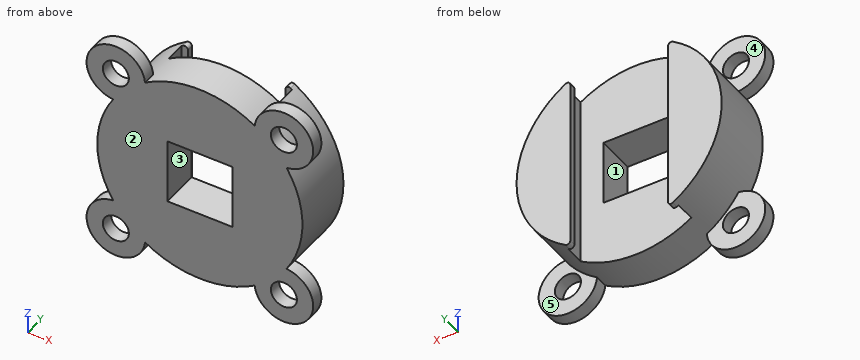
```python
from build123d import *

# Parameters (mm, degrees)
CYLINDER008_R         = 15.75
CYLINDER008_DEPTH     = 10
CYLINDER009_R         = 4.5
CYLINDER009_DEPTH     = 2
POLARPATTERN002_COUNT = 4
CYLINDER010_R         = 2
CYLINDER010_DEPTH     = 2
POLARPATTERN003_COUNT = 4
BOX001_W              = 10
BOX001_H              = 10
BOX001_DEPTH          = 10
BOX003_W              = 32.5
BOX003_H              = 17
BOX003_DEPTH          = 3.1
BOX004_W              = 32.5
BOX004_H              = 15
BOX004_DEPTH          = 1
FILLET005_R           = 0.5


with BuildPart() as part:
    # Cylinder008 → Cylinder008 (join)
    with BuildSketch(Plane(origin=(0, 0, 0), x_dir=(-1, 0, 0), z_dir=(0, 1, 0))):
        Circle(CYLINDER008_R)
    extrude(amount=CYLINDER008_DEPTH)

    # Cylinder009 → Cylinder009 (join)
    with BuildSketch(Plane(origin=(12.904699, 0, -12.904699), x_dir=(0, 0, -1), z_dir=(0, 1, 0))):
        Circle(CYLINDER009_R)
    cylinder009 = extrude(amount=CYLINDER009_DEPTH)

    # PolarPattern002: Cylinder009 ×4 about axis
    polarpattern002_axis = Axis((0, 0, 0), (0, 1, 0))
    for i in range(1, POLARPATTERN002_COUNT):
        add(cylinder009.rotate(polarpattern002_axis, i * 360 / POLARPATTERN002_COUNT))

    # Cylinder010 → Cylinder010 (cut)
    with BuildSketch(Plane(origin=(12.904699, 0, 12.904699), x_dir=(0, 0, -1), z_dir=(0, 1, 0))):
        Circle(CYLINDER010_R)
    cylinder010 = extrude(amount=CYLINDER010_DEPTH, mode=Mode.SUBTRACT)

    # PolarPattern003: Cylinder010 ×4 about axis
    polarpattern003_axis = Axis((0, 0, 0), (0, 1, 0))
    for i in range(1, POLARPATTERN003_COUNT):
        add(cylinder010.rotate(polarpattern003_axis, i * 360 / POLARPATTERN003_COUNT), mode=Mode.SUBTRACT)

    # Box001 → Box001 (cut)
    with BuildSketch(Plane(origin=(5, 0, -5), x_dir=(-1, 0, 0), z_dir=(0, 1, 0))):
        with Locations((5, 5)):
            Rectangle(BOX001_W, BOX001_H)
    extrude(amount=BOX001_DEPTH, mode=Mode.SUBTRACT)

    # Box003 → Box003 (cut)
    with BuildSketch(Plane(origin=(-8.5, 9, 16.25), x_dir=(0, 0, -1), z_dir=(0, -1, 0))):
        with Locations((16.25, 8.5)):
            Rectangle(BOX003_W, BOX003_H)
    extrude(amount=BOX003_DEPTH, mode=Mode.SUBTRACT)

    # Box004 → Box004 (cut)
    with BuildSketch(Plane(origin=(-7.5, 10, 16.25), x_dir=(0, 0, -1), z_dir=(0, -1, 0))):
        with Locations((16.25, 7.5)):
            Rectangle(BOX004_W, BOX004_H)
    extrude(amount=BOX004_DEPTH, mode=Mode.SUBTRACT)

    # Fillet005
    fillet005_edges = [part.edges().sort_by_distance(p)[0] for p in [
        (-7.5, 9.5, -13.849639),
        (7.5, 9.5, 13.849639),
        (-7.5, 9.5, 13.849639),
        (7.5, 9.5, -13.849639),
    ]]
    fillet(fillet005_edges, radius=FILLET005_R)


solid = part.part
```
Source: CAD feature listing. Evaluate the final solid. Frame: model axes, mm. Face numbers are marked on the shaded views. A direction names the side the tool comes from. Round coordinates to 2 decimals unless told otherwise and drop trailing zeros. Loops run counter-clockwise (first coordinate to the right, second up) from the corner with the lowest first, then second, coordinate; pieces in that order, holes last.
1. Mould query, pull axis Z, two halves, no side actions, for the marked faces 1 and 2. Classes: released by +Z, released by -Z, zero draft, split by the parting line, or undercut.
2. Ray query, L1, parallel to Y at x = -8, z = 11; L2, parallel to X at y = 1.75, z = -13.5; L3, parallel to X at y = 5.5, z = -2. Return the intervals inside material, ascending.
3. Access query for the marked faces 3, 4 and 5. Directions: +Z, -Z, +X, -X, +Y, -Y. A direction counts if a zero-diameter tool reaches every point of the face in a straight line with its end or side. Return the directions, or none.
4. Section query D-D on z = -11.5. Output: boundary loops of the cut face in (x, y), and give its area (3 significant figures).
5. Section query A-A on x = 0. Output: boundary loops of the cut face in (y, z).
6. Section query B-B on z = 0. Output: boundary loops of the cut face in (x, y).
7. Contact query for flat-ended pins moving along their axis: pin 1 (0.8 mm diameter, centred on y = 9.5, z = 0.5, fed in from -X); pin 2 (4.5 mm diameter, centred on x = 12.5, z = -13, fed in from +Y); pin 3 (1 mm diameter, centred on y = 8.5, z = 12, fed in from +X). Output: stop coordinate, or through.
8. Section query C-C on y = 8.5. Output: boundary loops of the cut face in (x, z), and give its area (3 significant figures).
Answers below:
1. face 1: undercut
1. face 2: zero draft
2. L1: y = 0 to 5.9, 9 to 10
2. L2: x = -17.37 to -14.81, -11 to -8.44, -8.11 to 8.11, 8.44 to 11, 14.81 to 17.37
2. L3: x = -15.62 to -5, 5 to 15.62
3. face 3: +Y, -Y
3. face 4: +Z, -X, +Y
3. face 5: -Z, +X, +Y
4. outline: (-17.18, 0) - (-14.33, 0) - (-14.33, 2) - (-17.18, 2) - close; (-11.48, 0) - (11.48, 0) - (11.48, 2) - (10.76, 2) - (10.76, 10) - (7.5, 10) - (7.5, 9) - (8.5, 9) - (8.5, 5.9) - (-8.5, 5.9) - (-8.5, 9) - (-7.5, 9) - (-7.5, 10) - (-10.76, 10) - (-10.76, 2) - (-11.48, 2) - close; (14.33, 0) - (17.18, 0) - (17.18, 2) - (14.33, 2) - close
4. area: 162 mm2
5. outline: (0, -15.75) - (5.9, -15.75) - (5.9, -5) - (0, -5) - close; (0, 5) - (5.9, 5) - (5.9, 15.75) - (0, 15.75) - close
6. outline: (-15.75, 0) - (-5, 0) - (-5, 5.9) - (-8.5, 5.9) - (-8.5, 9) - (-7.5, 9) - (-7.5, 10) - (-15.75, 10) - close; (5, 0) - (15.75, 0) - (15.75, 10) - (7.5, 10) - (7.5, 9) - (8.5, 9) - (8.5, 5.9) - (5, 5.9) - close
7. pin 1: stops at x = -15.75
7. pin 2: stops at y = 2
7. pin 3: stops at x = 10.76
8. outline: (-8.5, -13.26) - (-8.5, 13.26) arc R15.75 ccw to start; (8.5, -13.26) arc R15.75 ccw to (8.5, 13.26) - close
8. area: 271 mm2
